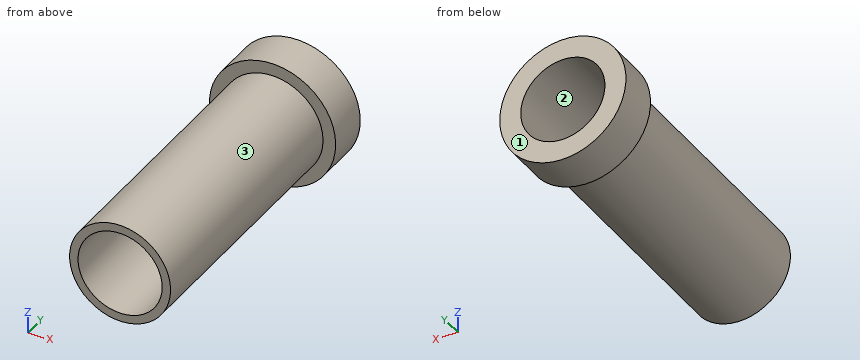
from build123d import *

# Parameters (mm, degrees)
ESQUISSE1_R      = 7.5
EXTRUSION1_DEPTH = 5
ESQUISSE2_R      = 6
EXTRUSION2_DEPTH = 31
EXTRUSION3_REACH = 38
ESQUISSE3_R      = 5


with BuildPart() as part:
    # Esquisse1 → Extrusion1 (new body)
    with BuildSketch(Plane(origin=(0, 0, 0), x_dir=(1, 0, 0), z_dir=(0, 1, 0))):
        Circle(ESQUISSE1_R)
    extrude(amount=EXTRUSION1_DEPTH)

    # Esquisse2 → Extrusion2 (add)
    with BuildSketch(Plane.XZ):
        Circle(ESQUISSE2_R)
    extrude(amount=EXTRUSION2_DEPTH)

    # Esquisse3 → Extrusion3 (cut, up to next)
    with BuildSketch(Plane(origin=(0, 5, 0), x_dir=(1, 0, 0), z_dir=(0, 1, 0)), mode=Mode.PRIVATE) as extrusion3_sk1:
        Circle(ESQUISSE3_R)
    extrusion3_tool1 = extrude(extrusion3_sk1.sketch, amount=-EXTRUSION3_REACH, mode=Mode.PRIVATE) & part.part
    add(extrusion3_tool1.solids().sort_by_distance((0, 5, 0))[0], mode=Mode.SUBTRACT)


solid = part.part
Input: part model. Units: mm. Frame: model coordinates. Face numbers are marked on the shaded views. Round coordinates to 2 decimals unless told otherwise and drop trailing zeros. Order: outer loops, then holes, each group sorted by start corner. A loop starts at its lowest first (then second) coordinate and runs counter-clockwise, first axis right, second up.
1. Cut plane A-A, the plane x = 0. Output: boundary loops of the cut face in (y, z).
The answers:
outline: (-31, -6) - (0, -6) - (0, -7.5) - (5, -7.5) - (5, -5) - (-31, -5) - close; (-31, 5) - (5, 5) - (5, 7.5) - (0, 7.5) - (0, 6) - (-31, 6) - close
2. Cut plane D-D, the plane x = -5.5. Output: boundary loops of the cut face in (y, z).
The answers:
outline: (-31, -2.4) - (0, -2.4) - (0, -5.1) - (5, -5.1) - (5, 5.1) - (0, 5.1) - (0, 2.4) - (-31, 2.4) - close
3. Material intervals for line 1 (Z direction, x = 0, y = -10.5); line 2 (X direction, y = -15, z = -1); line 3 (Y direction, x = 6, z = 3), sorted ascending.
The answers:
line 1: z = -6 to -5, 5 to 6
line 2: x = -5.92 to -4.9, 4.9 to 5.92
line 3: y = 0 to 5
4. Pin query (flat end, axial travel): P1, Ø4, axis at x = 2.5, y = -24, coming from the -Z side; P2, Ø1, axis at y = -1, z = 2, coming from the -X side; P3, Ø1, axis at x = 1.5, y = -17.5, coming from the +Z side; P4, Ø8, axis at x = 0, z = 0, coming from the -Y side. Return the tip coordinate at first contact, or that it passes through.
The answers:
P1: stops at z = -5.98
P2: stops at x = -5.81
P3: stops at z = 5.92
P4: passes through
5. Cut plane C-C, the plane y = -4. Output: boundary loops of the cut face in (x, z).
The answers:
outline: circle Ø12 at (0, 0); hole circle Ø10 at (0, 0)
6. Cut plane B-B, the plane z = 0. Output: boundary loops of the cut face in (x, y), then the cut area to 3 significant figures.
The answers:
outline: (-7.5, 0) - (-6, 0) - (-6, -31) - (-5, -31) - (-5, 5) - (-7.5, 5) - close; (5, -31) - (6, -31) - (6, 0) - (7.5, 0) - (7.5, 5) - (5, 5) - close
area: 87.0 mm2
7. Mould query, pull axis X, two halves, no side actions, for the marked faces 1, 2 and 3. Classes: released by +X, released by -X, zero draft, split by the parting line, or undercut.
The answers:
face 1: zero draft
face 2: undercut
face 3: split by the parting line
